```python
from build123d import *

# Parameters (mm, degrees)
SKETCH1_W           = 120
SKETCH1_H           = 60
BOSS_EXTRUDE1_DEPTH = 120
CUT_EXTRUDE1_DEPTH  = 120
CUT_EXTRUDE2_DEPTH  = 120
SKETCH5_R           = 40
CUT_EXTRUDE3_DEPTH  = 120


with BuildPart() as part:
    # Sketch1 → Boss-Extrude1 (new body)
    with BuildSketch(Plane.XY):
        with Locations((60, 30)):
            Rectangle(SKETCH1_W, SKETCH1_H)
    extrude(amount=BOSS_EXTRUDE1_DEPTH)

    # Sketch2 → Cut-Extrude1 (cut)
    with BuildSketch(Plane.XY.offset(120)):
        Polygon((0, 60), (0, 20), (10, 20), (10, 40), (90, 40), (90, 60), align=None)
    extrude(amount=-CUT_EXTRUDE1_DEPTH, mode=Mode.SUBTRACT)

    # Sketch3 → Cut-Extrude2 (cut)
    with BuildSketch(Plane(origin=(0, 0, 0), x_dir=(1, 0, 0), z_dir=(0, 1, 0))):
        with BuildLine():
            Line((120, 0), (60, 0))
            ThreePointArc((60, 0), (102.426406871, -17.573593129), (120, -60))
            Line((120, -60), (120, 0))
        make_face()
        with BuildLine():
            ThreePointArc((0, -60), (17.573593129, -17.573593129), (60, 0))
            Line((60, 0), (0, 0))
            Line((0, 0), (0, -60))
        make_face()
        with BuildLine():
            ThreePointArc((60, -120), (17.573593129, -102.426406871), (0, -60))
            Line((0, -60), (0, -120))
            Line((0, -120), (60, -120))
        make_face()
        with BuildLine():
            Line((120, -120), (120, -60))
            ThreePointArc((120, -60), (102.426406871, -102.426406871), (60, -120))
            Line((60, -120), (120, -120))
        make_face()
    extrude(amount=CUT_EXTRUDE2_DEPTH, mode=Mode.SUBTRACT)

    # Sketch5 → Cut-Extrude3 (cut)
    with BuildSketch(Plane(origin=(0, 0, 0), x_dir=(-1, 0, 0), z_dir=(0, -1, 0))):
        with Locations((-60, -60)):
            Circle(SKETCH5_R)
    extrude(amount=-CUT_EXTRUDE3_DEPTH, mode=Mode.SUBTRACT)


solid = part.part
```
Model file for the job. Use its own axes, mm. A direction names the side the tool comes from. Coordinates: 2 decimals unless noted, no trailing zeros. Order: outer loops, then holes, each group sorted by start corner. A loop starts at its lowest first (then second) coordinate and runs counter-clockwise, first axis right, second up. Notation, with made-up numbers: (-11.5, -11) -> (43.5, -11) arc R15 cw to (43.5, 15) -> close; hole circle Ø8 at (46, 78). An arc over 180 degrees is marked (long way). Return JSON: item names as keys, results as strings.
Item 1: Mould opens along Z. For faces 1 (the face through (90, 50, 21)), 2 (the face through (92, 23, 84)) say: pulls with the +Z half, pulls with the -Z half, needs draft (parallel to the pull), parting line crosses it, or undercut.
Model answer:
{"face 1": "needs draft", "face 2": "undercut"}
Item 2: Slice it at D-D (y = 48). Write the cut outline in (x, z).
Model answer:
{"outline": "(90, 8.04) arc R60 ccw to (90, 111.96) -> (90, 86.46) arc R40 cw to (90, 33.54) -> close"}
Item 3: Slice it at A-A (z = 52). Write the cut outline in (x, y).
Model answer:
{"outline": "(0.54, 0) -> (20.81, 0) -> (20.81, 40) -> (10, 40) -> (10, 20) -> (0.54, 20) -> close; (99.19, 0) -> (119.46, 0) -> (119.46, 60) -> (99.19, 60) -> close"}
Item 4: Slice it at B-B (x = 23.5). Write the cut outline in (y, z), then the cut area to 3 significant figures.
Model answer:
{"outline": "(0, 12.38) -> (40, 12.38) -> (40, 43.64) -> (0, 43.64) -> close; (0, 76.36) -> (40, 76.36) -> (40, 107.62) -> (0, 107.62) -> close", "area": "2,500 mm²"}
Item 5: 3-axis set-ups, long thin cutter, end or side, ignore diameter. For faces 3 (the face through (105, 60, 59)), 4 (the face through (6, 20, 60)): which of +Z, -Z, +X, -X, +Y, -Y reach the whole face in a straight line?
Model answer:
{"face 3": "+Z, -Z, +X, -X, +Y", "face 4": "+Z, -Z, -X, +Y"}
Item 6: Wall check: line 1 along Z through (x, y) = (60, 36); line 2 along X through (y, z) = (21, 60). Give the ranges that are in metal, low to high. Write a range as from..to.
Model answer:
{"line 1": "z = 0..20, 100..120", "line 2": "x = 10..20, 100..120"}
Item 7: Pin check, flat tips, straight feed: P1, Ø3, axis at x = 4.5, z = 46.5, coming from the +Y side; P2, Ø6, axis at y = 49.5, z = 27, coming from the -X side; P3, Ø2, axis at y = 26, z = 26.5, coming from the +X side. Stop position of each tip, or through.
Model answer:
{"P1": "stops at y = 20", "P2": "stops at x = 90", "P3": "stops at x = 110.44"}
Item 8: Slice it at C-C (y = 6). Write the cut outline in (x, z).
Model answer:
{"outline": "circle Ø120 at (60, 60); hole circle Ø80 at (60, 60)"}
